For this review, take the finished solid that the model builds, in its own axes (mm). A direction names the side the tool comes from. Round coordinates to 2 decimals unless told otherwise and drop trailing zeros. Loops run counter-clockwise (first coordinate to the right, second up) from the corner with the lowest first, then second, coordinate; pieces in that order, holes last.
1. Tool access review of faces 1 (the flat face through (-37.25, 4, -19)), 2 (the flat face through (15, 4, 15.5)), 3 (the flat face through (34, 4, 30)), 4 (the flat face through (21.5, 4, 25)): name each direction out of +Z, -Z, +X, -X, +Y, -Y from which nothing blocks a thin tool from reaching the whole face with its end or side.
2. Clearance check with a flat-ended pin moving along its axis: pin 1 Ø1 at (x, y) = (19, 3) entering from +Z. State where the tip first meets the part, or that it passes through.
3. Consider section A-A on z = 0.5. State the section outline as (x, y) points.
4. Consider section C-C on z = -18. State the section outline as (x, y) points, then the cut area to 3 significant figures.
5. Consider section D-D on x = -30. State the section outline as (y, z) points.
6. Consider section B-B on x = -40. State the section outline as (y, z) points, then the cut area to 3 significant figures.
7. To check wall thickness, follow line 1 along X through (y, z) = (4.25, -15.5); line 2 along Z through (x, y) = (-10, 1); line 3 along X through (y, z) = (3, 22). State the ranges of each line that lie inside material, in increasing order.
8. Draft analysis for pull direction Z (two halves, no side actions). For faces 5 (the cylindrical face through (30, 4, 28)), 6 (the flat face through (-34, 4, 30)), 7 (the flat face through (-13, 7, 18)), 8 (the flat face through (31.75, 4, 18)), state which applies: released by +Z, released by -Z, zero draft, split by the parting line, or undercut.
from build123d import *

# Parameters (mm, degrees)
SKETCH1_W           = 30
SKETCH1_H           = 15
BOSS_EXTRUDE1_DEPTH = 8
SKETCH4_R           = 6.45
CUT_EXTRUDE1_DEPTH  = 11
CUT_EXTRUDE2_DEPTH  = 5.5
CHAMFER1_SIZE       = 2
FILLET1_R           = 3


with BuildPart() as part:
    # Sketch1 → Boss-Extrude1 (new body)
    with BuildSketch(Plane(origin=(0, 0, 0), x_dir=(1, 0, 0), z_dir=(0, 1, 0))):
        Polygon((50, 30), (-50, 30), (-50, -30), (-21.5, -30), (-21.5, -21), (-18, -21), (-18, -15.5), (-13, -15.5), (-13, -21), (-11.5, -21), (-11.5, -18.5), (11.5, -18.5), (11.5, -21), (13, -21), (13, -15.5), (18, -15.5), (18, -21), (21.5, -21), (21.5, -30), (50, -30), align=None)
        with BuildLine():
            ThreePointArc((-42.75, -15), (-40, -12.25), (-37.25, -15))
            Line((-37.25, -15), (-37.25, -19))
            Line((-37.25, -19), (-37.25, -23))
            ThreePointArc((-37.25, -23), (-40, -25.75), (-42.75, -23))
            Line((-42.75, -23), (-42.75, -19))
            Line((-42.75, -19), (-42.75, -15))
        make_face(mode=Mode.SUBTRACT)
        with BuildLine():
            ThreePointArc((-28.25, -26.25), (-30, -28), (-31.75, -26.25))
            Line((-31.75, -26.25), (-31.75, -10.81))
            ThreePointArc((-31.75, -10.81), (-30, -9.06), (-28.25, -10.81))
            Line((-28.25, -10.81), (-28.25, -26.25))
        make_face(mode=Mode.SUBTRACT)
        with BuildLine():
            ThreePointArc((28.25, -10.81), (30, -9.06), (31.75, -10.81))
            Line((31.75, -10.81), (31.75, -26.25))
            ThreePointArc((31.75, -26.25), (30, -28), (28.25, -26.25))
            Line((28.25, -26.25), (28.25, -10.81))
        make_face(mode=Mode.SUBTRACT)
        with BuildLine():
            ThreePointArc((42.75, -23), (40, -25.75), (37.25, -23))
            Line((37.25, -23), (37.25, -19))
            Line((37.25, -19), (37.25, -15))
            ThreePointArc((37.25, -15), (40, -12.25), (42.75, -15))
            Line((42.75, -15), (42.75, -19))
            Line((42.75, -19), (42.75, -23))
        make_face(mode=Mode.SUBTRACT)
        with BuildLine():
            ThreePointArc((-42.75, 23), (-40, 25.75), (-37.25, 23))
            Line((-37.25, 23), (-37.25, 19))
            Line((-37.25, 19), (-37.25, 15))
            ThreePointArc((-37.25, 15), (-40, 12.25), (-42.75, 15))
            Line((-42.75, 15), (-42.75, 19))
            Line((-42.75, 19), (-42.75, 23))
        make_face(mode=Mode.SUBTRACT)
        Rectangle(SKETCH1_W, SKETCH1_H, mode=Mode.SUBTRACT)
        with BuildLine():
            ThreePointArc((37.25, 23), (40, 25.75), (42.75, 23))
            Line((42.75, 23), (42.75, 19))
            Line((42.75, 19), (42.75, 15))
            ThreePointArc((42.75, 15), (40, 12.25), (37.25, 15))
            Line((37.25, 15), (37.25, 19))
            Line((37.25, 19), (37.25, 23))
        make_face(mode=Mode.SUBTRACT)
    extrude(amount=BOSS_EXTRUDE1_DEPTH)

    # Sketch4 → Cut-Extrude1 (cut)
    with BuildSketch(Plane.XY.offset(18.5)):
        with Locations((0, 8)):
            Circle(SKETCH4_R)
    extrude(amount=-CUT_EXTRUDE1_DEPTH, mode=Mode.SUBTRACT)

    # Sketch5 → Cut-Extrude2 (cut)
    with BuildSketch(Plane.XY.offset(21)):
        Polygon((13, 0), (13, 5.2), (11.5, 1.5), (11.5, 0), align=None)
        Polygon((19.75, 0), (18, 2), (18, 0), align=None)
        Polygon((-11.5, 0), (-11.5, 1.5), (-13, 5.2), (-13, 0), align=None)
        Polygon((-18, 2), (-19.75, 0), (-18, 0), align=None)
        Polygon((11.5, 0), (11.5, 1.5), (10.5, 0), align=None)
        Polygon((-11.5, 0), (-10.5, 0), (-11.5, 1.5), align=None)
    extrude(amount=-CUT_EXTRUDE2_DEPTH, mode=Mode.SUBTRACT)

    # Chamfer1
    chamfer1_edges = [part.edges().sort_by_distance(p)[0] for p in [
        (50, 8, 0),
        (0, 8, -30),
        (-50, 8, 0),
    ]]
    chamfer(chamfer1_edges, length=CHAMFER1_SIZE)

    # Fillet1
    fillet1_edges = [part.edges().sort_by_distance(p)[0] for p in [
        (-50, 3, 30),
        (50, 3, 30),
        (50, 3, -30),
        (-50, 3, -30),
    ]]
    fillet(fillet1_edges, radius=FILLET1_R)


solid = part.part
Resolved:
1. face 1: +Y, -Y
1. face 2: +Z, -Y
1. face 3: +Z, +X, -X, +Y, -Y
1. face 4: +Z, +Y, -Y
2. pin 1: stops at z = 21
3. outline: (-50, 0) - (-15, 0) - (-15, 8) - (-48, 8) - (-50, 6) - close; (15, 0) - (50, 0) - (50, 6) - (48, 8) - (15, 8) - close
4. outline: (-50, 0) - (-42.75, 0) - (-42.75, 8) - (-48, 8) - (-50, 6) - close; (-37.25, 0) - (37.25, 0) - (37.25, 8) - (-37.25, 8) - close; (42.75, 0) - (50, 0) - (50, 6) - (48, 8) - (42.75, 8) - close
4. area: 708 mm2
5. outline: (0, -30) - (6, -30) - (8, -28) - (8, 9.06) - (0, 9.06) - close; (0, 28) - (8, 28) - (8, 30) - (0, 30) - close
6. outline: (0, -30) - (6, -30) - (8, -28) - (8, -25.75) - (0, -25.75) - close; (0, -12.25) - (8, -12.25) - (8, 12.25) - (0, 12.25) - close; (0, 25.75) - (8, 25.75) - (8, 30) - (0, 30) - close
6. area: 262 mm2
7. line 1: x = -50 to -42.75, -37.25 to 37.25, 42.75 to 50
7. line 2: z = -30 to -7.5, 7.5 to 18.5
7. line 3: x = -50 to -42.75, -37.25 to -31.75, -28.25 to -21.5, 21.5 to 28.25, 31.75 to 37.25, 42.75 to 50
8. face 5: undercut
8. face 6: released by +Z
8. face 7: zero draft
8. face 8: undercut
